```python
from build123d import *

# Parameters (mm, degrees)
EXTRUDE_1_DEPTH       = 16
CUT_EXTRUDE_1_DEPTH   = 13
CUT_EXTRUDE_1_2_DEPTH = 3.5
CUT_EXTRUDE_2_DEPTH   = 14.5


with BuildPart() as part:
    # Model → Extrude 1 (new body)
    # profile 1 of 3: a face of its own
    with BuildSketch(Plane.XY):
        Polygon((375.566, -7.74368854), (-7.904930268, -7.726795577), (-7.935386074, 184.294), (375.473711158, 184.294), align=None)
        Polygon((367.76326137, 176.494), (367.76600301, 0.079153109), (-0.110128346, 0.072857135), (-0.101373388, 176.494), align=None, mode=Mode.SUBTRACT)
    # profile 2 of 3: a face of its own
    with BuildSketch(Plane.XY):
        Polygon((367.76600301, 0.079153109), (-0.110128346, 0.072857135), (-0.101373388, 176.494), (367.76326137, 176.494), align=None)
        Polygon((359.870508087, 168.593), (359.86752, 7.972254), (7.7946046, 7.972254), (7.787335087, 168.593), align=None, mode=Mode.SUBTRACT)
    # profile 3 of 3: a face of its own
    with BuildSketch(Plane.XY):
        Polygon((359.86752, 7.972254), (7.7946046, 7.972254), (7.787335087, 168.593), (359.870508087, 168.593), align=None)
    extrude(amount=EXTRUDE_1_DEPTH)

    # Sketch 3 → Cut-Extrude 1 (cut)
    # profile 1 of 2: a face of its own
    with BuildSketch(Plane.XY.offset(16)):
        Polygon((-6.404930287, -7.726557667), (-6.435386093, 184.29423791), (-4.935386112, 184.29447582), (-4.904930306, -7.726319757), align=None)
    # profile 2 of 2: a face of its own
    with BuildSketch(Plane.XY.offset(16)):
        Polygon((375.473711158, 184.294), (-7.935386074, 184.294), (-7.904930268, -7.726795577), (375.566, -7.74368854), align=None)
        Polygon((373.97443185, 182.794), (-6.435148145, 182.794), (-6.405168149, -6.226861644), (374.06527893, -6.243622428), align=None, mode=Mode.SUBTRACT)
    extrude(amount=-CUT_EXTRUDE_1_DEPTH, mode=Mode.SUBTRACT)

    # Sketch 3_5 → Cut-Extrude 1 2 (cut)
    with BuildSketch(Plane.XY.offset(16)):
        Polygon((-6.435148145, 182.794), (-6.405168149, -6.226861644), (374.06527893, -6.243622428), (373.97443185, 182.794), align=None)
    extrude(amount=-CUT_EXTRUDE_1_2_DEPTH, mode=Mode.SUBTRACT)

    # Sketch 4 → Cut-Extrude 2 (cut)
    with BuildSketch(Plane.XY.offset(12.5)):
        Polygon((7.7946046, 7.972254), (359.86752, 7.972254), (359.870508087, 168.593), (7.787335087, 168.593), align=None)
    extrude(amount=-CUT_EXTRUDE_2_DEPTH, mode=Mode.SUBTRACT)


solid = part.part
```
CAD build for the part. Positions are in the model's coordinates, mm. A direction names the side the tool comes from. Give positions to 0.01 mm unless a question says otherwise; leave off trailing zeros. Write each loop counter-clockwise with the first axis right and the second up, starting at its lowest first coordinate (ties: lowest second). Pieces come first, ordered by that corner, then holes. Notation, with made-up numbers: (-20.5, 85.5) -> (38.5, 85.5) arc R26 cw to (38.5, 107.5) -> close; hole circle Ø7 at (-3, 2). An arc over 180 degrees is marked (long way). Write each question's results on one line, items separated by ' | '.
1. Wall check: probe 1 along Y at (x, z) = (71, 7); probe 2 along X at (y, z) = (67.5, 9.5); probe 3 along Y at (x, z) = (50, 1.5). Give the ranges that are in metal, low to high. Write a range as [from, to].
Geometry check:
probe 1: [-6.23, 7.97], [168.59, 182.79] | probe 2: [-4.92, 7.79], [359.87, 374.03] | probe 3: [-7.73, 7.97], [168.59, 184.29]
2. Cut at B-B, the plane x = 315. Write the cut outline in (y, z), then the cut area to 3 significant figures.
Geometry check:
outline: (-7.74, 0) -> (7.97, 0) -> (7.97, 12.5) -> (-6.24, 12.5) -> (-6.24, 3) -> (-7.74, 3) -> close; (168.59, 0) -> (184.29, 0) -> (184.29, 3) -> (182.79, 3) -> (182.79, 12.5) -> (168.59, 12.5) -> close | area: 364 mm²
3. Drop flat-ended pins along their axis: P1, Ø1, axis at y = 69.5, z = 5.5, coming from the -X side; P2, Ø6, axis at x = 117.5, z = 8, coming from the -Y side; P3, Ø7.5, axis at x = 247.5, z = 10, coming from the +Y side. Give the stop position or say it passes through.
Geometry check:
P1: x = -4.92 | P2: y = -6.23 | P3: y = 182.79
4. Two-plate mould, pull along X, no slides. Class faces 1 (the flat face through (170, 5, 12.5)), 2 (the flat face through (181, 7.972, 6)): pulls with the +X half, pulls with the -X half, needs draft (parallel to the pull), parting line crosses it, or undercut.
Geometry check:
face 1: needs draft | face 2: undercut
5. Cut at A-A, the plane z = 7.25. Write the cut outline in (x, y).
Geometry check:
outline: (-4.94, 182.79) -> (-4.91, -6.23) -> (374.07, -6.24) -> (373.97, 182.79) -> close; hole (7.79, 7.97) -> (359.87, 7.97) -> (359.87, 168.59) -> (7.79, 168.59) -> close
6. Cut at C-C, the plane y = 111. Write the cut outline in (x, z), then the cut area to 3 significant figures.
Geometry check:
outline: (-7.92, 0) -> (7.79, 0) -> (7.79, 12.5) -> (-4.92, 12.5) -> (-4.92, 3) -> (-7.92, 3) -> close; (359.87, 0) -> (375.51, 0) -> (375.51, 3) -> (374.01, 3) -> (374.01, 12.5) -> (359.87, 12.5) -> close | area: 349 mm²
7. Which spindle directions (+Z, -Z, +X, -X, +Y, -Y) get a long thin tool onto all of the face, cutting with end or side? Do faces 3 (the flat face through (199, 3, 0)), 4 (the flat face through (187, 182.794, 8)), 5 (the flat face through (186, 168.593, 6)). Say none if no direction does.
Geometry check:
face 3: -Z, +X, -X, +Y, -Y | face 4: +Z, +X, -X, +Y | face 5: +Z, -Z
